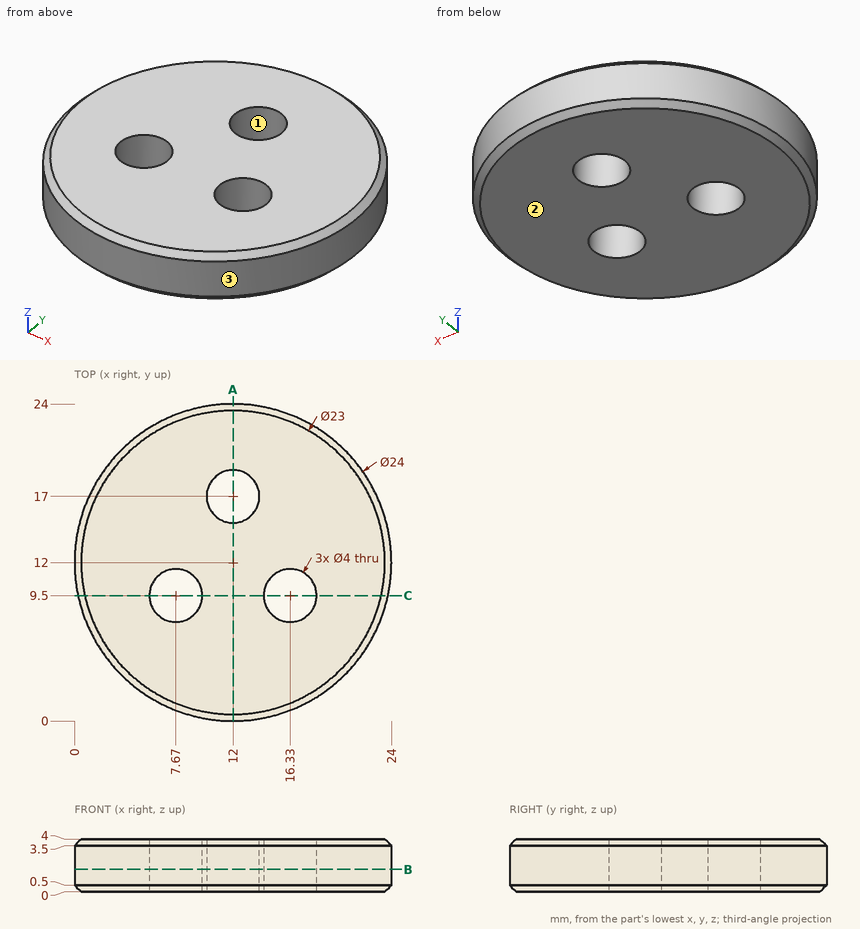
Verification items for this drawing (mm, ordinates from the low corner). Coordinates: 2 decimals unless noted, no trailing zeros. Write each loop counter-clockwise with the first axis right and the second up, starting at its lowest first coordinate (ties: lowest second). Pieces come first, ordered by that corner, then holes. Notation, with made-up numbers: (-16.5, 31.5) -> (1.5, 31.5) arc R36 cw to (1.5, 67.5) -> close; hole circle Ø7 at (-22, -34.5). An arc over 180 degrees is marked (long way). One line per item, written item: value. Start each with the question number.
Q1. Cross-section at C-C on y = 9.5. State how many separate pieces and enclosed holes the cut face has, and give its area (3 significant figures).
Q2. Mould release check, pull along X, two halves, no side actions. Record for the marked faces 1, 2 and 3: pulls with the +X half, pulls with the -X half, needs draft (parallel to the pull), parting line crosses it, or undercut.
Q3. Cross-section at B-B on z = 1.7. Enter the section's corners in (x, y), and give its area (3 significant figures).
Q4. Cross-section at A-A on x = 12. Enter the section's corners in (y, z).
Q5. Thickness scan on L1, parallel to X at y = 10.25, z = 2.9; L2, parallel to X at y = 17.25, z = 3.45; L3, parallel to X at y = 18.25, z = 0.3. Record the ranges inside material, lowest first. Write a range as from..to.
Q6. Go/stop test with flat-tipped pins: P1, Ø2, axis at y = 18, z = 3, coming from the -X side; P2, Ø3.5, axis at x = 16.33, y = 9.5, coming from the -Z side; P3, Ø1.5, axis at x = 5, z = 1.5, coming from the -Y side. Record where each tip stops, or that it passes through.
Checked values:
1. separate pieces: 3
1. enclosed holes: 0
1. area: 61.4 mm²
2. face 1: undercut
2. face 2: needs draft
2. face 3: parting line crosses it
3. outline: circle Ø24 at (12, 12); hole circle Ø4 at (7.67, 9.5); hole circle Ø4 at (12, 17); hole circle Ø4 at (16.33, 9.5)
3. area: 415 mm²
4. outline: (0, 0.5) -> (0.5, 0) -> (15, 0) -> (15, 4) -> (0.5, 4) -> (0, 3.5) -> close; (19, 0) -> (23.5, 0) -> (24, 0.5) -> (24, 3.5) -> (23.5, 4) -> (19, 4) -> close
5. L1: x = 0.13..5.82, 9.52..14.48, 18.18..23.87
5. L2: x = 1.21..10.02, 13.98..22.79
5. L3: x = 1.99..10.44, 13.56..22.01
6. P1: stops at x = 1.09
6. P2: passes through
6. P3: stops at y = 1.76
